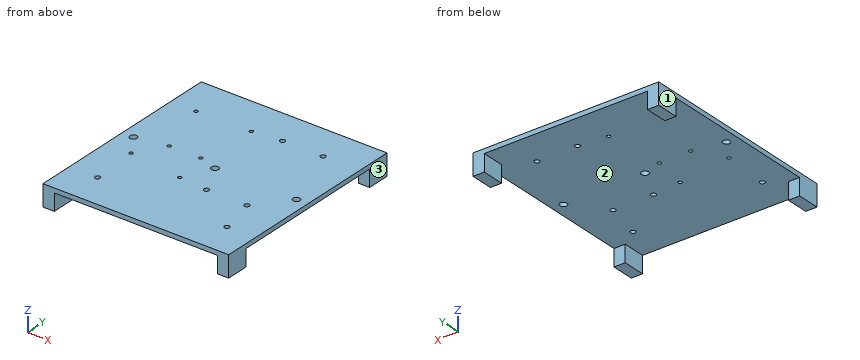
```python
from build123d import *

# Parameters (mm, degrees)
SKETCH1_W           = 165
SKETCH1_H           = 182.31
BOSS_EXTRUDE1_DEPTH = 4
SKETCH2_R           = 2.2
SKETCH2_R_2         = 1.6
CUT_EXTRUDE1_DEPTH  = 4
SKETCH3_W           = 10
SKETCH3_H           = 20
BOSS_EXTRUDE2_DEPTH = 15
CUT_EXTRUDE2_REACH  = 175.429
SKETCH4_R           = 3.1


with BuildPart() as part:
    # Sketch1 → Boss-Extrude1 (new body)
    with BuildSketch(Plane.XY):
        with Locations((0, 60.655)):
            Rectangle(SKETCH1_W, SKETCH1_H)
    extrude(amount=BOSS_EXTRUDE1_DEPTH)

    # Sketch2 → Cut-Extrude1 (cut)
    with BuildSketch(Plane(origin=(0, 0, 0), x_dir=(-1, 0, 0), z_dir=(0, 0, -1))):
        with Locations((-49.884295567, 120.4)):
            Circle(SKETCH2_R)
        with Locations((-49.884295567, 32.9)):
            Circle(SKETCH2_R)
        with Locations((-13.884295567, 32.9)):
            Circle(SKETCH2_R)
        with Locations((-13.884295567, 120.4)):
            Circle(SKETCH2_R)
        with Locations((57.5, 0)):
            Circle(SKETCH2_R)
        with Locations((-57.5, 0)):
            Circle(SKETCH2_R)
        with Locations((11.655704433, 35.29)):
            Circle(SKETCH2_R_2)
        with Locations((16.815704433, 66)):
            Circle(SKETCH2_R_2)
        with Locations((11.655704433, 117.69)):
            Circle(SKETCH2_R_2)
        with Locations((59.915704433, 116.57)):
            Circle(SKETCH2_R_2)
        with Locations((44.715704433, 66)):
            Circle(SKETCH2_R_2)
        with Locations((59.915704433, 41.64)):
            Circle(SKETCH2_R_2)
    extrude(amount=-CUT_EXTRUDE1_DEPTH, mode=Mode.SUBTRACT)

    # Sketch3 → Boss-Extrude2 (add)
    with BuildSketch(Plane(origin=(0, 0, 0), x_dir=(-1, 0, 0), z_dir=(0, 0, -1))):
        with Locations((-77.5, -20.5)):
            Rectangle(SKETCH3_W, SKETCH3_H)
        with Locations((-77.5, 141.81)):
            Rectangle(SKETCH3_W, SKETCH3_H)
        with Locations((77.5, -20.5)):
            Rectangle(SKETCH3_W, SKETCH3_H)
        with Locations((77.5, 141.81)):
            Rectangle(SKETCH3_W, SKETCH3_H)
    extrude(amount=BOSS_EXTRUDE2_DEPTH)

    # Sketch4 → Cut-Extrude2 (cut, up to next)
    with BuildSketch(Plane(origin=(0, 0, 0), x_dir=(-1, 0, 0), z_dir=(0, 0, -1)), mode=Mode.PRIVATE) as cut_extrude2_sk1:
        with Locations((-72.5, 60.655)):
            Circle(SKETCH4_R)
    cut_extrude2_tool1 = extrude(cut_extrude2_sk1.sketch, amount=-CUT_EXTRUDE2_REACH, mode=Mode.PRIVATE) & part.part
    # Sketch4 → Cut-Extrude2 (cut, up to next)
    with BuildSketch(Plane(origin=(0, 0, 0), x_dir=(-1, 0, 0), z_dir=(0, 0, -1)), mode=Mode.PRIVATE) as cut_extrude2_sk2:
        with Locations((72.5, 60.655)):
            Circle(SKETCH4_R)
    cut_extrude2_tool2 = extrude(cut_extrude2_sk2.sketch, amount=-CUT_EXTRUDE2_REACH, mode=Mode.PRIVATE) & part.part
    # Sketch4 → Cut-Extrude2 (cut, up to next)
    with BuildSketch(Plane(origin=(0, 0, 0), x_dir=(-1, 0, 0), z_dir=(0, 0, -1)), mode=Mode.PRIVATE) as cut_extrude2_sk3:
        with Locations((0, 60.655)):
            Circle(SKETCH4_R)
    cut_extrude2_tool3 = extrude(cut_extrude2_sk3.sketch, amount=-CUT_EXTRUDE2_REACH, mode=Mode.PRIVATE) & part.part
    add(cut_extrude2_tool1.solids().sort_by_distance((72.5, 60.655, 0))[0], mode=Mode.SUBTRACT)
    add(cut_extrude2_tool2.solids().sort_by_distance((-72.5, 60.655, 0))[0], mode=Mode.SUBTRACT)
    add(cut_extrude2_tool3.solids().sort_by_distance((0, 60.655, 0))[0], mode=Mode.SUBTRACT)


solid = part.part
```
Input: part model. Units: mm. Frame: model coordinates. Face numbers are marked on the shaded views. Give positions to 0.01 mm unless a question says otherwise; leave off trailing zeros. Order: outer loops, then holes, each group sorted by start corner. A loop starts at its lowest first (then second) coordinate and runs counter-clockwise, first axis right, second up. Notation, with made-up numbers: (-38.5, -26.75) - (-29.5, -26.75) arc R25 ccw to (-29.5, -0.75) - close; hole circle Ø11 at (73, -14.5). An arc over 180 degrees is marked (long way). One line per item, written item: value.
1. Pin query (flat end, axial travel): pin 1 Ø3.5 at (x, y) = (-11.66, 35.29) entering from -Z; pin 2 Ø10 at (x, y) = (-72.5, 60.655) entering from +Z. Return the tip coordinate at first contact, or that it passes through.
Determined:
pin 1: z = 0
pin 2: z = 4
2. Line query: probe 1 along X at (y, z) = (66, 2.85); probe 2 along X at (y, z) = (117.69, 1.9); probe 3 along Y at (x, z) = (0, 0.8) (3 decimals). Output: solid intervals per line, ascending.
Determined:
probe 1: -82.5 to -46.32, -43.12 to -18.42, -15.22 to 82.5
probe 2: -82.5 to -61.06, -58.77 to -13.26, -10.06 to 82.5
probe 3: -30.5 to 57.555, 63.755 to 151.81
3. Cut plane C-C, the plane y = 0. Output: boundary loops of the cut face in (x, z), and give its area (3 significant figures).
Determined:
outline: (-82.5, 0) - (-59.7, 0) - (-59.7, 4) - (-82.5, 4) - close; (-55.3, 0) - (55.3, 0) - (55.3, 4) - (-55.3, 4) - close; (59.7, 0) - (82.5, 0) - (82.5, 4) - (59.7, 4) - close
area: 625 mm2
4. Cut plane D-D, the plane y = 134.5. Output: boundary loops of the cut face in (x, z), and give its area (3 significant figures).
Determined:
outline: (-82.5, -15) - (-72.5, -15) - (-72.5, 0) - (72.5, 0) - (72.5, -15) - (82.5, -15) - (82.5, 4) - (-82.5, 4) - close
area: 960 mm2
5. Cut plane B-B, the plane z = -6. Output: boundary loops of the cut face in (x, y), and give its area (3 significant figures).
Determined:
outline: (-82.5, -30.5) - (-72.5, -30.5) - (-72.5, -10.5) - (-82.5, -10.5) - close; (-82.5, 131.81) - (-72.5, 131.81) - (-72.5, 151.81) - (-82.5, 151.81) - close; (72.5, -30.5) - (82.5, -30.5) - (82.5, -10.5) - (72.5, -10.5) - close; (72.5, 131.81) - (82.5, 131.81) - (82.5, 151.81) - (72.5, 151.81) - close
area: 800 mm2
6. Draft query along X for the marked faces 1, 2 and 3. Return one class per face: released by +X, released by -X, zero draft, split by the parting line, or undercut.
Determined:
face 1: released by -X
face 2: undercut
face 3: released by +X
7. Cut plane A-A, the plane x = 0. Output: boundary loops of the cut face in (y, z) (3 decimals), and give its area (3 significant figures).
Determined:
outline: (-30.5, 0) - (57.555, 0) - (57.555, 4) - (-30.5, 4) - close; (63.755, 0) - (151.81, 0) - (151.81, 4) - (63.755, 4) - close
area: 704 mm2
